CAD build for the part. Positions are in the model's coordinates, mm. Coordinates: 2 decimals unless noted, no trailing zeros. Order: outer loops, then holes, each group sorted by start corner. A loop starts at its lowest first (then second) coordinate and runs counter-clockwise, first axis right, second up. Notation, with made-up numbers: M 34.25,43 L 87.25,43 A30 cw 87.25,72 Z; hole C 37,-28.75 d2. An arc over 180 degrees is marked long. One line per item, written item: value.
from build123d import *

# Parameters (mm, degrees)
EXTRUDE_1_DEPTH     = 5.2
SKETCH_5_R          = 3
CUT_EXTRUDE_1_DEPTH = 10.239769118


with BuildPart() as part:
    # Sketch 1 → Extrude 1 (new body)
    with BuildSketch(Plane.XY):
        Polygon((0, 5.773502692), (-5, 2.886751346), (-5, -2.886751346), (0, -5.773502692), (5, -2.886751346), (5, 2.886751346), align=None)
    extrude(amount=EXTRUDE_1_DEPTH)

    # Sketch 4 → Cut-Revolve 1 (revolve, cut)
    with BuildSketch(Plane(origin=(0, 0, 0), x_dir=(0, 0, -1), z_dir=(1, 0, 0)), mode=Mode.PRIVATE) as cut_revolve_1_sk:
        Polygon((-5.2, -4.5), (-4.736482927, -5.773502692), (-5.2, -5.773502692), align=None)
    cut_revolve_1 = revolve(cut_revolve_1_sk.sketch.rotate(Axis((0, 0, 5.2), (0, 0, -1)), 119.999999979), axis=Axis((0, 0, 5.2), (0, 0, -1)), mode=Mode.SUBTRACT)

    # Mirror 1: Cut-Revolve 1 across plane
    add(cut_revolve_1.mirror(Plane.XY.offset(2.6)), mode=Mode.SUBTRACT)

    # Sketch 5 → Cut-Extrude 1 (cut, through all)
    with BuildSketch(Plane.XY.offset(5.2)):
        Circle(SKETCH_5_R)
    extrude(amount=-CUT_EXTRUDE_1_DEPTH, mode=Mode.SUBTRACT)


solid = part.part
Q1. Pin check, flat tip, straight feed: pin 1 Ø1.5 at (x, z) = (-3.5, 1) entering from -Y. Stop position of the tip, or through.
Recorded:
pin 1: stops at y = -4.19
Q2. Mould opens along X. For faces 1 (the face through (-2.465, 4.35, 2.566)), 2 (the face through (2.465, -4.35, 2.566)), 3 (the face through (-3, 0, 3)) say: released by +X, released by -X, zero draft, split by the parting line, or undercut.
Recorded:
face 1: released by -X
face 2: released by +X
face 3: undercut
Q3. Drill centre lines: line 1 along X through (y, z) = (-1.5, 1.3); line 2 along X through (y, z) = (-1.25, 4.5); line 3 along Y through (x, z) = (0.25, 1.3). Where is each one in solid material? Low to high.
Recorded:
line 1: x = -5 to -2.6, 2.6 to 5
line 2: x = -5 to -2.73, 2.73 to 5
line 3: y = -5.63 to -2.99, 2.99 to 5.63
Q4. Slice it at A-A (y = 0). List the corners of the cut face in (x, z), plus the area to 3 significant figures.
Recorded:
outline: M -5,0.18 L -4.5,0 L -3,0 L -3,5.2 L -4.5,5.2 L -5,5.02 Z; M 3,0 L 4.5,0 L 5,0.18 L 5,5.02 L 4.5,5.2 L 3,5.2 Z
area: 20.6 mm^2
Q5. Slice it at B-B (z = 2.8). List the corners of the cut face in (x, y).
Recorded:
outline: M -5,-2.89 L 0,-5.77 L 5,-2.89 L 5,2.89 L 0,5.77 L -5,2.89 Z; hole C 0,0 d6
